Could you check a few things on this model? Use its own coordinates, in mm. Round coordinates to 2 decimals unless told otherwise and drop trailing zeros. Loops run counter-clockwise (first coordinate to the right, second up) from the corner with the lowest first, then second, coordinate; pieces in that order, holes last. Notation, with made-up numbers: M 3,32.25 L 24,32.25 A20 ccw 24,63.25 Z; hole C 65,44.5 d9. An arc over 180 degrees is marked long. Answer in a Markdown table with one row per item.
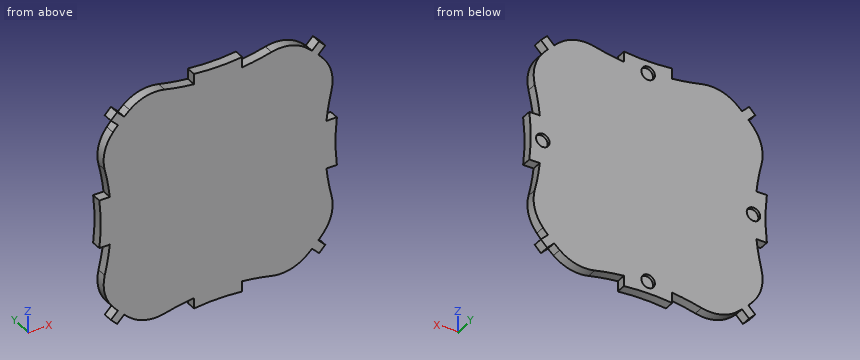
```python
from build123d import *

# Parameters (mm, degrees)
SKETCH1_R                = 35.433
BOSS_EXTRUDE1_DEPTH      = 2.54
SKETCH2_R                = 59.158135963
CUT_EXTRUDE1_DEPTH       = 51.174162454
BOSS_EXTRUDE3_DEPTH      = 2.54
SKETCH4_R                = 1.7399
CUT_EXTRUDE2_DEPTH       = 0.762
FILLET1_R                = 10.287
EXTRUDE_THIN1_DEPTH      = 2.54
CIRPATTERN1_COUNT        = 4
FILLET1_OF_CIRPATTERN1_R = 10.287


with BuildPart() as part:
    # Sketch1 → Boss-Extrude1 (new body)
    with BuildSketch(Plane(origin=(0, 0, 0), x_dir=(1, 0, 0), z_dir=(0, 1, 0))):
        with Locations(Location((0, 0, 0), (0, 0, 270))):
            Circle(SKETCH1_R)
    extrude(amount=BOSS_EXTRUDE1_DEPTH)

    # Sketch2 → Cut-Extrude1 (cut, through all)
    with BuildSketch(Plane(origin=(0, 2.54, 0), x_dir=(1, 0, 0), z_dir=(0, 1, 0))):
        with Locations((0, 86.777928127)):
            Circle(SKETCH2_R)
    cut_extrude1 = extrude(amount=-CUT_EXTRUDE1_DEPTH, mode=Mode.SUBTRACT)

    # Sketch3 → Boss-Extrude3 (add)
    with BuildSketch(Plane(origin=(0, 0, 0), x_dir=(-1, 0, 0), z_dir=(0, -1, 0))):
        with BuildLine():
            Line((6.223, 22.34125112), (-6.223, 22.34125112))
            Line((-6.223, 22.34125112), (-6.223, 30.630597706))
            ThreePointArc((-6.223, 30.630597706), (0, 30.286792164), (6.223, 30.630597706))
            Line((6.223, 30.630597706), (6.223, 22.34125112))
        make_face()
    boss_extrude3 = extrude(amount=-BOSS_EXTRUDE3_DEPTH)

    # Sketch4 → Cut-Extrude2 (cut)
    with BuildSketch(Plane(origin=(0, 2.54, 0), x_dir=(1, 0, 0), z_dir=(0, 1, 0))):
        with Locations(Location((0, 27.178, 0), (0, 0, 270))):
            Circle(SKETCH4_R)
    cut_extrude2 = extrude(amount=-CUT_EXTRUDE2_DEPTH, mode=Mode.SUBTRACT)

    # Fillet1
    fillet1_edges = [part.edges().sort_by_distance(p)[0] for p in [
        (18.104908895, 1.27, -30.458328301),
        (-18.104908895, 1.27, -30.458328301),
    ]]
    fillet(fillet1_edges, radius=FILLET1_R)

    # Sketch5 → Extrude-Thin1 (add)
    with BuildSketch(Plane(origin=(0, 2.54, 0), x_dir=(1, 0, 0), z_dir=(0, 1, 0))):
        Polygon((0.808223051, -0.808223051), (27.659188853, 26.042742751), (26.042742751, 27.659188853), (-0.808223051, 0.808223051), align=None)
    extrude_thin1 = extrude(amount=-EXTRUDE_THIN1_DEPTH)

    # CirPattern1: Cut-Extrude1, Boss-Extrude3, Cut-Extrude2, Extrude-Thin1 ×4 about axis
    cirpattern1_axis = Axis((0, 0, 0), (0, 1, 0))
    add([cut_extrude1.rotate(cirpattern1_axis, i * 360 / CIRPATTERN1_COUNT) for i in range(1, CIRPATTERN1_COUNT)], mode=Mode.SUBTRACT)
    add([boss_extrude3.rotate(cirpattern1_axis, i * 360 / CIRPATTERN1_COUNT) for i in range(1, CIRPATTERN1_COUNT)])
    add([cut_extrude2.rotate(cirpattern1_axis, i * 360 / CIRPATTERN1_COUNT) for i in range(1, CIRPATTERN1_COUNT)], mode=Mode.SUBTRACT)
    add([extrude_thin1.rotate(cirpattern1_axis, i * 360 / CIRPATTERN1_COUNT) for i in range(1, CIRPATTERN1_COUNT)])

    # Fillet1 of CirPattern1
    fillet1_of_cirpattern1_edges = [part.edges().sort_by_distance(p)[0] for p in [
        (-30.458328301, 1.27, -18.104908895),
        (-30.458328301, 1.27, 18.104908895),
        (-18.104908895, 1.27, 30.458328301),
        (18.104908895, 1.27, 30.458328301),
        (30.458328301, 1.27, 18.104908895),
        (30.458328301, 1.27, -18.104908895),
    ]]
    fillet(fillet1_of_cirpattern1_edges, radius=FILLET1_OF_CIRPATTERN1_R)


solid = part.part
```
1) I want a section at A-A, the plane z = 0. Please give me the cut outline in (x, y), plus the area to 3 significant figures.
Computed:
| item | result |
|---|---|
| outline | M -30.29,0 L 30.29,0 L 30.29,2.54 L 28.92,2.54 L 28.92,1.78 L 25.44,1.78 L 25.44,2.54 L -25.44,2.54 L -25.44,1.78 L -28.92,1.78 L -28.92,2.54 L -30.29,2.54 Z |
| area | 149 mm² |
2) I want a section at B-B, the plane x = 0. Please give me the cut outline in (y, z).
Computed:
| item | result |
|---|---|
| outline | M 0,-30.29 L 2.54,-30.29 L 2.54,-28.92 L 1.78,-28.92 L 1.78,-25.44 L 2.54,-25.44 L 2.54,25.44 L 1.78,25.44 L 1.78,28.92 L 2.54,28.92 L 2.54,30.29 L 0,30.29 Z |
3) Will these pins go through, and if not, where does the flat tip stop? P1, Ø1.5, axis at y = 0.5, z = -23.5, coming from the -X side; P2, Ø1.5, axis at x = 23, y = 2, coming from the -Z side; P3, Ø3, axis at x = 0, z = -27.178, coming from the +Y side.
Computed:
| item | result |
|---|---|
| P1 | stops at x = -27.16 |
| P2 | stops at z = -27.55 |
| P3 | stops at y = 1.78 |
4) I need wall thicknesses on line 1 (Z direction, x = -16.5, y = 0.3); line 2 (X direction, y = 1.55, z = 17.5). Which ranges of each line are inside material? Lowest first, please.
Computed:
| item | result |
|---|---|
| line 1 | z = -29.53 to 29.53 |
| line 2 | x = -29.45 to 29.45 |
